Verification items for the finished model (mm, model axes). A direction names the side the tool comes from. Give positions to 0.01 mm unless a question says otherwise; leave off trailing zeros. Order: outer loops, then holes, each group sorted by start corner. A loop starts at its lowest first (then second) coordinate and runs counter-clockwise, first axis right, second up.
from build123d import *

# Parameters (mm, degrees)
F1_DEPTH       = 30
F2_W           = 73
F2_H           = 21
F3_DEPTH       = 5
F4_W           = 73
F4_H           = 110
F5_DEPTH       = 3
F9_DEPTH       = 15
F12_DEPTH      = 20
F13_W          = 20
F13_H          = 15
F14_DEPTH      = 15
F16_DEPTH      = 20
F17_R          = 1.5
F18_DEPTH      = 49.4
F19_W          = 10
F19_H          = 11
F20_DEPTH      = 10.001
F21_W          = 15
F21_H          = 12
F22_DEPTH      = 46.501
F24_DEPTH      = 10
F25_R          = 2.25
F26_DEPTH      = 10.55
F28_DEPTH      = 10
F28_DEPTH_BACK = 2


with BuildPart() as f1:
    # F0 (on Top) → F1 (new body)
    with BuildSketch(Plane.XY):
        Polygon((-36.5, -21), (-18.5, -21), (-18.5, -18), (-33.5, -18), (-33.5, -3), (33.5, -3), (33.5, -18), (18.5, -18), (18.5, -21), (36.5, -21), (36.5, 0), (-36.5, 0), align=None)
    extrude(amount=F1_DEPTH)

    # F2 (on Top) → F3 (join)
    with BuildSketch(Plane.XY):
        with Locations((0, -10.5)):
            Rectangle(F2_W, F2_H)
    extrude(amount=F3_DEPTH)

    # F4 (on Front) → F5 (join)
    with BuildSketch(Plane.XZ):
        with Locations((0, 85)):
            Rectangle(F4_W, F4_H)
    extrude(amount=F5_DEPTH)

    # F8 (on offset) → F9 (join)
    with BuildSketch(Plane.XY.offset(60)):
        Polygon((-18.5, -18), (-33.5, -18), (-33.5, -3), (-36.5, -3), (-36.5, -21), (-18.5, -21), align=None)
        Polygon((33.5, -18), (18.5, -18), (18.5, -21), (36.5, -21), (36.5, -3), (33.5, -3), align=None)
    extrude(amount=F9_DEPTH)

    # F11 (on offset) → F12 (join)
    with BuildSketch(Plane.XY.offset(140)):
        Polygon((-33.5, -18), (-33.5, -3), (-36.5, -3), (-36.5, -21), (-18.5, -21), (-18.5, -18), align=None)
        Polygon((36.5, -21), (36.5, -3), (33.5, -3), (33.5, -18), (18.5, -18), (18.5, -21), align=None)
    extrude(amount=-F12_DEPTH)

    # F13 (on offset) → F14 (join)
    with BuildSketch(Plane.XY.offset(60)):
        with Locations((0, 7.5)):
            Rectangle(F13_W, F13_H)
    extrude(amount=F14_DEPTH)

    # F15 (on face) → F16 (join)
    with BuildSketch(Plane.YZ.offset(10)):
        with BuildLine():
            ThreePointArc((37, 64), (26, 53), (15, 64))
            Line((15, 64), (13, 64))
            ThreePointArc((13, 64), (24.502876321, 51.0864946397), (38.6551724138, 61.0256746686))
            ThreePointArc((38.6551724138, 61.0256746686), (43.5583407717, 65.7019258868), (37, 64))
        make_face()
    extrude(amount=-F16_DEPTH)

    # F17 (on face) → F18 (cut)
    with BuildSketch(Plane.YZ.offset(10)):
        with Locations((40.5, 64)):
            Circle(F17_R)
    extrude(amount=-F18_DEPTH, mode=Mode.SUBTRACT)

    # F19 (on offset) → F20 (cut, through all)
    with BuildSketch(Plane.XZ.offset(-34)):
        with Locations((0, 65.5)):
            Rectangle(F19_W, F19_H)
    extrude(amount=-F20_DEPTH, mode=Mode.SUBTRACT)

    # F21 (on face) → F22 (cut, through all)
    with BuildSketch(Plane(origin=(-10, 0, 0), x_dir=(0, -1, 0), z_dir=(-1, 0, 0))):
        with Locations((-9.5, 70)):
            Rectangle(F21_W, F21_H)
    extrude(amount=-F22_DEPTH, mode=Mode.SUBTRACT)

    # F23 (on Right) → F24 (join, symmetric)
    with BuildSketch(Plane.YZ):
        Polygon((0, 56.2852394792), (0, 50.3416226459), (8.7014795803, 60), (3.3467229155, 60), align=None)
    extrude(amount=F24_DEPTH, both=True)

    # F25 (on offset) → F26 (cut, symmetric)
    with BuildSketch(Plane.XY.offset(60)):
        with Locations((0, 9)):
            Circle(F25_R)
    extrude(amount=F26_DEPTH, both=True, mode=Mode.SUBTRACT)

    # F27 (on face) → F28 (cut, two sides)
    with BuildSketch(Plane.XY.offset(60)) as f28_sk:
        Polygon((2.1650635095, 5.25), (4.3301270189, 9), (2.1650635095, 12.75), (-2.1650635095, 12.75), (-4.3301270189, 9), (-2.1650635095, 5.25), align=None)
    extrude(amount=-F28_DEPTH, mode=Mode.SUBTRACT)
    extrude(f28_sk.sketch, amount=F28_DEPTH_BACK, mode=Mode.SUBTRACT)


solid = f1.part
(1) Set-up check for faces 1 (the flat face through (10, 15, 61)), 2 (the flat face through (0, 2, 69)), 3 (the flat face through (34, -15, 30)), 4 (the flat face through (26, -18, 17)): record each of +Z, -Z, +X, -X, +Y, -Y from which the full face is reachable in a straight line by a thin tool's end or side.
Solved:
face 1: +Z, -Z, +X, +Y
face 2: +Z, +X, -X
face 3: +X, -X, -Y
face 4: +Z
(2) Go/stop test with flat-tipped pins: pin 1 (8 mm diameter, centred on x = 13.5, y = -14, fed in from -Z); pin 2 (9 mm diameter, centred on x = 9.5, y = -12, fed in from +Z); pin 3 (0.6 mm diameter, centred on x = -1, y = 37, fed in from +Z); pin 4 (5.5 mm diameter, centred on x = -2, z = 69, fed in from +Y). Record where each tip stops, or that it passes through.
Solved:
pin 1: stops at z = 0
pin 2: stops at z = 5
pin 3: stops at z = 60
pin 4: stops at y = 2
(3) Section check A-A, the plane x = 21.5. Enter the section's corners in (y, z).
Solved:
outline: (-21, 0) - (0, 0) - (0, 140) - (-3, 140) - (-3, 5) - (-18, 5) - (-18, 30) - (-21, 30) - close; (-21, 60) - (-18, 60) - (-18, 75) - (-21, 75) - close; (-21, 120) - (-18, 120) - (-18, 140) - (-21, 140) - close
(4) Release check for a two-part mould opening along Y. For faces 5 (the flat face through (5, 39, 63)), 6 (the cylindrical face through (-0.29, 11.23, 63.01)), 7 (the flat face through (27, -21, 130)) record: pulls with the +Y half, pulls with the -Y half, needs draft (parallel to the pull), parting line crosses it, or undercut.
Solved:
face 5: needs draft
face 6: undercut
face 7: pulls with the -Y half
(5) Section check C-C, the plane x = 0. Enter the section's corners in (y, z).
Solved:
outline: (-21, 0) - (0, 0) - (0, 50.34) - (5.25, 56.17) - (5.25, 62) - (6.75, 62) - (6.75, 64) - (2, 64) - (2, 75) - (0, 75) - (0, 140) - (-3, 140) - (-3, 5) - (-21, 5) - close; (11.25, 62) - (12.75, 62) - (12.75, 60) - (13.63, 60) arc R13 ccw to (38.37, 60) - (36.25, 60) arc R11 cw to (15, 64) - (11.25, 64) - close; hole (0, 56.29) - (3.35, 60) - (0, 60) - close
(6) Section check D-D, the plane z = 125.5. Enter the section's corners in (x, y), then the cut area to 3 significant figures.
Solved:
outline: (-36.5, -21) - (-18.5, -21) - (-18.5, -18) - (-33.5, -18) - (-33.5, -3) - (33.5, -3) - (33.5, -18) - (18.5, -18) - (18.5, -21) - (36.5, -21) - (36.5, 0) - (-36.5, 0) - close
area: 417 mm2
(7) Section check B-B, the plane y = 40.5. Enter the section's corners in (x, z).
Solved:
outline: (-10, 60.5) - (-5, 60.5) - (-5, 62.5) - (-10, 62.5) - close; (-10, 65.5) - (-5, 65.5) - (-5, 67.5) - (-10, 67.5) - close; (5, 60.5) - (10, 60.5) - (10, 62.5) - (5, 62.5) - close; (5, 65.5) - (10, 65.5) - (10, 67.5) - (5, 67.5) - close
(8) Scan lines: line 1 (X direction, y = -6, z = 120.5); line 2 (Y direction, x = -24, z = 72); line 3 (Y direction, x = -20.5, z = 101). Record each from-to range of solid material in increasing order.
Solved:
line 1: x = -36.5 to -33.5, 33.5 to 36.5
line 2: y = -21 to -18, -3 to 0
line 3: y = -3 to 0
